Can you work these out from the model? Positions are in its coordinate system, mm. Face numbers are marked on the shaded views. A direction names the side the tool comes from. Round coordinates to 2 decimals unless told otherwise and drop trailing zeros. Loops run counter-clockwise (first coordinate to the right, second up) from the corner with the lowest first, then second, coordinate; pieces in that order, holes last.
```python
from build123d import *

# Parameters (mm, degrees)
BOSS_EXTRUDE1_DEPTH      = 25.4
BOSS_EXTRUDE1_DEPTH_BACK = 34.925
CUT_EXTRUDE4_DEPTH       = 63.941922635
CUT_EXTRUDE5_DEPTH       = 46.01339384
SKETCH14_R               = 3.2893
CUT_EXTRUDE6_DEPTH       = 46.01339384
CUT_EXTRUDE7_DEPTH       = 38.1
CUT_EXTRUDE7_DEPTH_BACK  = 25.4
SKETCH15_R               = 12.7
CUT_EXTRUDE21_DEPTH      = 14.732
CUT_EXTRUDE21_DEPTH_BACK = 25.4
SKETCH16_R               = 12.7
CUT_EXTRUDE22_DEPTH      = 16.51
CUT_EXTRUDE22_DEPTH_BACK = 12.7
SKETCH17_R               = 12.7
CUT_EXTRUDE23_DEPTH      = 16.51
CUT_EXTRUDE23_DEPTH_BACK = 12.7
SKETCH18_R               = 12.7
CUT_EXTRUDE24_DEPTH      = 12.7
CUT_EXTRUDE24_DEPTH_BACK = 12.7
SKETCH19_R               = 12.7
SKETCH20_W               = 58.413051364
SKETCH20_H               = 40.891520134
CUT_EXTRUDE25_DEPTH      = 51.98499249


with BuildPart() as part:
    # Sketch1 → Boss-Extrude1 (new, two sides: drawn at the far end of the back side and taken through both)
    with BuildSketch(Plane(origin=(0, 0, 0), x_dir=(0, 0, -1), z_dir=(1, 0, 0)).offset(-BOSS_EXTRUDE1_DEPTH_BACK)):
        with BuildLine():
            Line((-10.16, 12.7), (10.16, 12.7))
            ThreePointArc((10.16, 12.7), (11.956051224, 11.956051224), (12.7, 10.16))
            Line((12.7, 10.16), (12.7, -10.16))
            ThreePointArc((12.7, -10.16), (11.956051224, -11.956051224), (10.16, -12.7))
            Line((10.16, -12.7), (-10.16, -12.7))
            ThreePointArc((-10.16, -12.7), (-11.956051224, -11.956051224), (-12.7, -10.16))
            Line((-12.7, -10.16), (-12.7, 10.16))
            ThreePointArc((-12.7, 10.16), (-11.956051224, 11.956051224), (-10.16, 12.7))
        make_face()
    extrude(amount=BOSS_EXTRUDE1_DEPTH + BOSS_EXTRUDE1_DEPTH_BACK)

    # Sketch11 → Cut-Extrude4 (cut, through all)
    with BuildSketch(Plane(origin=(25.4, 0, 0), x_dir=(0, 0, -1), z_dir=(1, 0, 0))):
        with BuildLine():
            Line((-10.6045, 11.1125), (10.6045, 11.1125))
            ThreePointArc((10.6045, 11.1125), (10.963710245, 10.963710245), (11.1125, 10.6045))
            Line((11.1125, 10.6045), (11.1125, -10.6045))
            ThreePointArc((11.1125, -10.6045), (10.963710245, -10.963710245), (10.6045, -11.1125))
            Line((10.6045, -11.1125), (-10.6045, -11.1125))
            ThreePointArc((-10.6045, -11.1125), (-10.963710245, -10.963710245), (-11.1125, -10.6045))
            Line((-11.1125, -10.6045), (-11.1125, 10.6045))
            ThreePointArc((-11.1125, 10.6045), (-10.963710245, 10.963710245), (-10.6045, 11.1125))
        make_face()
    extrude(amount=-CUT_EXTRUDE4_DEPTH, mode=Mode.SUBTRACT)

    # Sketch12 → Cut-Extrude5 (cut, through all)
    with BuildSketch(Plane(origin=(0, 12.7, 0), x_dir=(1, 0, 0), z_dir=(0, 1, 0))):
        with BuildLine():
            Line((0, 12.7), (50.8, 12.7))
            Line((50.8, 12.7), (50.8, -12.7))
            Line((50.8, -12.7), (0, -12.7))
            Line((0, -12.7), (19.444424463, -7.686083637))
            ThreePointArc((19.444424463, -7.686083637), (25.4, 0), (19.444424463, 7.686083637))
            Line((19.444424463, 7.686083637), (0, 12.7))
        make_face()
    extrude(amount=-CUT_EXTRUDE5_DEPTH, mode=Mode.SUBTRACT)

    # Sketch14 → Cut-Extrude6 (cut, through all)
    with BuildSketch(Plane(origin=(0, 12.7, 0), x_dir=(1, 0, 0), z_dir=(0, 1, 0))):
        with Locations(Location((17.4625, 0, 0), (0, 0, 270))):
            Circle(SKETCH14_R)
    extrude(amount=-CUT_EXTRUDE6_DEPTH, mode=Mode.SUBTRACT)

    # Sketch15 → Cut-Extrude7 (cut, two sides: drawn at the far end of the back side and taken through both)
    with BuildSketch(Plane(origin=(-18.580944095, -12.7, 0.022320862), x_dir=(0.966128643141705, 0.25805311522873825, -0.0020086368292127157), z_dir=(-0.2580609325356477, 0.9660993767043436, -0.007519935525706381)).offset(-CUT_EXTRUDE7_DEPTH_BACK)):
        with Locations(Location((0, 0, 0), (0, 0, 51.828658107))):
            Circle(SKETCH15_R)
    extrude(amount=CUT_EXTRUDE7_DEPTH + CUT_EXTRUDE7_DEPTH_BACK, mode=Mode.SUBTRACT)

    # Sketch16 → Cut-Extrude21 (cut, two sides: drawn at the far end of the back side and taken through both)
    with BuildSketch(Plane(origin=(-34.925, -13.993557422, 0), x_dir=(0, 0, -1), z_dir=(0.9661266940476224, 0.2580682294444863, 0)).offset(-CUT_EXTRUDE21_DEPTH_BACK)):
        Circle(SKETCH16_R)
    extrude(amount=CUT_EXTRUDE21_DEPTH + CUT_EXTRUDE21_DEPTH_BACK, mode=Mode.SUBTRACT)

    # Sketch17 → Cut-Extrude22 (cut, two sides: drawn at the far end of the back side and taken through both)
    with BuildSketch(Plane(origin=(-29.427114325, -12.623836713, -12.7), x_dir=(0.7903344181486555, -0.13152541034589554, -0.5983916559603502), z_dir=(0.6126756952006717, 0.1696640808045107, 0.7719084092009455)).offset(-CUT_EXTRUDE22_DEPTH_BACK)):
        Circle(SKETCH17_R)
    extrude(amount=CUT_EXTRUDE22_DEPTH + CUT_EXTRUDE22_DEPTH_BACK, mode=Mode.SUBTRACT)


with BuildPart() as cut_extrude22_piece_1:
    # of the separate pieces the step leaves, piece 1, a body of its own (cut_extrude22_pieces)
    add(part.part.solids().sort_by_distance((-34.925, 10.16, 12.7))[0])


with BuildPart() as cut_extrude22_piece_2:
    # of the separate pieces the step leaves, piece 2, a body of its own (cut_extrude22_pieces)
    add(part.part.solids().sort_by_distance((-28.657579441, 0.553532164, -11.1125))[0])


with BuildPart() as cut_extrude23_tool:
    # Sketch18 → Cut-Extrude23 (new, two sides: drawn at the far end of the back side and taken through both)
    with BuildSketch(Plane(origin=(-17.958929348, -9.56049708, -12.7), x_dir=(0.9940833845942288, -0.002324974713650623, 0.10859474649477009), z_dir=(-0.10861963208224606, -0.02127809391484378, 0.9938556324968274)).offset(-CUT_EXTRUDE23_DEPTH_BACK)):
        Circle(SKETCH18_R)
    extrude(amount=CUT_EXTRUDE23_DEPTH + CUT_EXTRUDE23_DEPTH_BACK)


with BuildPart() as cut_extrude22_piece_1_1:
    add(cut_extrude22_piece_1.part)

    # Cut-Extrude23: cut by cut_extrude23_tool
    add(cut_extrude23_tool.part, mode=Mode.SUBTRACT)

    # Sketch19 → Cut-Extrude24 (cut, two sides: drawn at the far end of the back side and taken through both)
    with BuildSketch(Plane(origin=(-16.211316351, -16.081156217, -12.7), x_dir=(0.9763290145154149, 0.09548845507502933, 0.1940711476823458), z_dir=(-0.21629067343590844, 0.43103175814295297, 0.8760308031438372)).offset(-CUT_EXTRUDE24_DEPTH_BACK)):
        Circle(SKETCH19_R)
    extrude(amount=CUT_EXTRUDE24_DEPTH + CUT_EXTRUDE24_DEPTH_BACK, mode=Mode.SUBTRACT)


with BuildPart() as cut_extrude22_piece_2_1:
    add(cut_extrude22_piece_2.part)

    # Cut-Extrude23: cut by cut_extrude23_tool
    add(cut_extrude23_tool.part, mode=Mode.SUBTRACT)


with BuildPart() as cut_extrude25_tool:
    # Sketch20 → Cut-Extrude25 (new, through all)
    with BuildSketch(Plane(origin=(-20.509915766, -5.478533696, 0), x_dir=(0.25806093253564766, -0.9660993767043435, 0.007519935525706381), z_dir=(0.9661266940476224, 0.2580682294444864, 0))):
        Rectangle(SKETCH20_W, SKETCH20_H)
    extrude(amount=-CUT_EXTRUDE25_DEPTH)


with BuildPart() as cut_extrude22_piece_1_2:
    add(cut_extrude22_piece_1_1.part)

    # Cut-Extrude25: cut by cut_extrude25_tool
    add(cut_extrude25_tool.part, mode=Mode.SUBTRACT)


with BuildPart() as cut_extrude22_piece_2_2:
    add(cut_extrude22_piece_2_1.part)

    # Cut-Extrude25: cut by cut_extrude25_tool
    add(cut_extrude25_tool.part, mode=Mode.SUBTRACT)


solid = cut_extrude22_piece_1_2.part
```
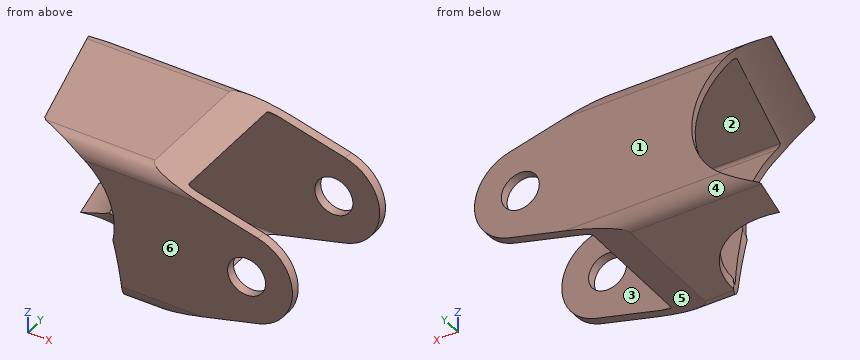
(1) If I drill on line 1 (Y direction, x = 8, z = -8.5); line 2 (Z direction, x = 4.5, y = -8), over which ranges is the centre line in solid material (lowest first)?
(2) For pin 1 (2 mm diameter, centred on y = 3.5, z = -8.5, fed in from +X); pin 2 (10 mm diameter, centred on x = 8, y = 3.5, fed in from -Z), each with a flat end and sliding along its axis, tell me the tip position at first contact or that it passes through.
(3) Suppose I cut it at C-C (z = 0). Give the number of separate pieces and of enclosed holes in the cut face, then the cut area to 3 significant figures.
(4) We'd pull the mould along Y, two halves only. Please class the marked faces 3, 4, 5 and 6: released by +Y, released by -Y, zero draft, split by the parting line, or undercut.
(5) Suppose I cut it at A-A (x = -0.5). Write out the boundary of the cut face in (y, z).
(6) Suppose I cut it at B-B (x = 20). Write out the boundary of the cut face in (y, z), then the cut area to 3 significant figures.
(7) Which directions (+Z, -Z, +X, -X, +Y, -Y) give clear straight access to the entire face, cutting with the end or side of a thin tool? Please do the marked faces 1 and 2.
Check result:
1. line 1: y = -12.7 to -11.11, 11.11 to 12.7
1. line 2: z = -11.54 to -11.11, 11.11 to 11.54
2. pin 1: passes through
2. pin 2: stops at z = -11.93
3. separate pieces: 4
3. enclosed holes: 0
3. area: 87.8 mm2
4. face 3: undercut
4. face 4: released by +Y
4. face 5: zero draft
4. face 6: released by -Y
5. outline: (-12.7, -10.16) arc R2.54 ccw to (-10.16, -12.7) - (10.16, -12.7) arc R2.54 ccw to (12.7, -10.16) - (12.7, 10.16) arc R2.54 ccw to (10.16, 12.7) - (-10.16, 12.7) arc R2.54 ccw to (-12.7, 10.16) - close; hole (-11.11, -10.6) arc R0.51 ccw to (-10.6, -11.11) - (10.6, -11.11) arc R0.51 ccw to (11.11, -10.6) - (11.11, 10.6) arc R0.51 ccw to (10.6, 11.11) - (-10.6, 11.11) arc R0.51 ccw to (-11.11, 10.6) - close
6. outline: (-12.7, -7.52) - (-11.11, -7.52) - (-11.11, -2.09) - (-12.7, -2.09) - close; (-12.7, 2.09) - (-11.11, 2.09) - (-11.11, 7.52) - (-12.7, 7.52) - close; (11.11, -7.52) - (12.7, -7.52) - (12.7, -2.09) - (11.11, -2.09) - close; (11.11, 2.09) - (12.7, 2.09) - (12.7, 7.52) - (11.11, 7.52) - close
6. area: 34.5 mm2
7. face 1: +Z, -Z, +X, -X, +Y
7. face 2: +X, -X
